from build123d import *

# Parameters (mm, degrees)
REDONDEO1_R           = 10
CROQUIS4_R            = 1.65
CORTAR_EXTRUIR1_DEPTH = 5
CORTAR_EXTRUIR2_DEPTH = 2


with BuildPart() as part:
    # Croquis1 → Revolución3 (revolve)
    with BuildSketch(Plane.XY):
        Polygon((-20, -5), (-20, 100), (0, 123), (0, 120), (-17, 100), (-17, 0), (-10, 0), (-10, -5), align=None)
    revolve(axis=Axis((0, 0, 0), (0, 1, 0)))

    # Redondeo1
    redondeo1_edges = [part.edges().sort_by_distance(p)[0] for p in [
        (20, 100, 0),
    ]]
    fillet(redondeo1_edges, radius=REDONDEO1_R)

    # Croquis4 → Cortar-Extruir1 (cut)
    with BuildSketch(Plane.XZ.offset(5)):
        with Locations((12.5, 0)):
            Circle(CROQUIS4_R)
        with Locations((-12.5, 0)):
            Circle(CROQUIS4_R)
    extrude(amount=-CORTAR_EXTRUIR1_DEPTH, mode=Mode.SUBTRACT)

    # Croquis5 → Cortar-Extruir2 (cut)
    with BuildSketch(Plane(origin=(0, 0, 0), x_dir=(1, 0, 0), z_dir=(0, 1, 0))):
        Polygon((-12.5, 3.4), (-15.444486373, 1.7), (-15.444486373, -1.7), (-12.5, -3.4), (-9.555513627, -1.7), (-9.555513627, 1.7), align=None)
        Polygon((12.5, 3.4), (9.555513627, 1.7), (9.555513627, -1.7), (12.5, -3.4), (15.444486373, -1.7), (15.444486373, 1.7), align=None)
    extrude(amount=-CORTAR_EXTRUIR2_DEPTH, mode=Mode.SUBTRACT)


solid = part.part
Model file for the job. Use its own axes, mm. A direction names the side the tool comes from. Give positions to 0.01 mm unless a question says otherwise; leave off trailing zeros. Loops run counter-clockwise (first coordinate to the right, second up) from the corner with the lowest first, then second, coordinate; pieces in that order, holes last.
1) Tool access for faces 4 (the cylindrical face through (-19.076, 46.339, 6.007)), 5 (the flat face through (13, -2, -2)), 6 (the cylindrical face through (-10.976, -3.521, -0.632)): list every direction of +Z, -Z, +X, -X, +Y, -Y with a clear straight run to the whole face (end or side of a thin tool).
2) Saw through at B-B (y = 106.5). Write the cut outline in (x, z) (3 decimals), plus the area to 3 significant figures.
3) Saw through at A-A (y = 50.5). Write the cut outline in (x, z), plus the area to 3 significant figures.
4) Pull direction Y, two halves, no side cores. Call faces 1 (the conical face through (-4.53, 117.54, 1.43)), 2 (the flat face through (-5, -5, 9)), 3 (the flat face through (-7.3, 0, -7.3)): +Y half, -Y half, draft (parallel to the pull), parting line (faces both ways), or undercut.
5) Flat gauge pins, fed straight in: pin 1 Ø5 at (x, y) = (-10, 108.5) entering from -Z; pin 2 Ø1.7 at (x, z) = (12.5, -0.5) entering from +Y; pin 3 Ø3 at (x, z) = (7.5, 7.5) entering from +Y. Where does each tip first touch, or does it go through?
6) Wall check: line 1 (X direction, y = 16.5, z = 0.5); line 2 (X direction, y = -1.8, z = 0); line 3 (Z direction, x = 0, y = -3.85). Give the ranges that are in metal, low to high.
Answer block:
1. face 4: +Y, -Y
1. face 5: none
1. face 6: -Y
2. outline: circle Ø28.696 at (0, 0); hole circle Ø22.95 at (0, 0)
2. area: 233 mm2
3. outline: circle Ø40 at (0, 0); hole circle Ø34 at (0, 0)
3. area: 349 mm2
4. face 1: +Y half
4. face 2: -Y half
4. face 3: undercut
5. pin 1: stops at z = -11.56
5. pin 2: stops at y = 109.59
5. pin 3: stops at y = 112.53
6. line 1: x = -19.99 to -16.99, 16.99 to 19.99
6. line 2: x = -20 to -15.44, 15.44 to 20
6. line 3: z = -20 to -10, 10 to 20
